Can you work these out from the model? Positions are in its coordinate system, mm. A direction names the side the tool comes from. Give positions to 0.01 mm unless a question says otherwise; leave off trailing zeros. Order: outer loops, then holes, each group sorted by start corner. A loop starts at its lowest first (then second) coordinate and runs counter-clockwise, first axis right, second up. Notation, with made-up numbers: M 2,88.5 L 46,88.5 A22 cw 46,104.5 Z; hole C -19.5,56.25 d10. An arc over 180 degrees is marked long. Use a Markdown table: item, result. Add a question column.
from build123d import *

# Parameters (mm, degrees)
SKETCH4_R                = 6.35
BOSS_EXTRUDE1_DEPTH      = 6.35
BOSS_EXTRUDE1_DEPTH_BACK = 6.35
SKETCH5_R                = 6.35
SKETCH5_R_2              = 5.9436
CUT_EXTRUDE1_DEPTH       = 1.4224
SKETCH7_W                = 1.89865
SKETCH7_H                = 6.35


with BuildPart() as part:
    # Sketch4 → Boss-Extrude1 (new body, two sides)
    with BuildSketch(Plane.XY.offset(39.04234)) as boss_extrude1_sk:
        with Locations((-94.293901082, 0)):
            Circle(SKETCH4_R)
    extrude(amount=BOSS_EXTRUDE1_DEPTH)
    extrude(boss_extrude1_sk.sketch, amount=-BOSS_EXTRUDE1_DEPTH_BACK)

    # Sketch5 → Cut-Extrude1 (cut)
    with BuildSketch(Plane.XY.offset(34.44494)):
        with Locations((-94.293901082, 0)):
            Circle(SKETCH5_R)
        with Locations((-94.293901082, 0)):
            Circle(SKETCH5_R_2, mode=Mode.SUBTRACT)
    extrude(amount=CUT_EXTRUDE1_DEPTH, mode=Mode.SUBTRACT)

    # Sketch7 → Tap Drill for _10-24 Tap1 (revolve, cut)
    with BuildSketch(Plane(origin=(-94.293901082, 0, 39.04234), x_dir=(0, 1, 0), z_dir=(1, 0, 0))):
        with Locations((0.949325, 3.175)):
            Rectangle(SKETCH7_W, SKETCH7_H)
    revolve(axis=Axis((-94.293901082, 0, 32.69234), (0, 0, 1)), mode=Mode.SUBTRACT)


solid = part.part
1. If we section it at D-D, the plane z = 42.75: List the corners of the cut face in (x, y) for me.
2. I need wall thicknesses on L1, parallel to Z at x = -95.5, y = 1; L2, parallel to X at y = 0.5, z = 41; L3, parallel to Y at x = -95, z = 41.5. Which ranges of each line are inside material? Lowest first, please. Write a range as [from, to].
3. Will these pins go through, and if not, where does the flat tip stop? pin 1 (3 mm diameter, centred on x = -98.5, y = -5, fed in from -Z); pin 2 (1 mm diameter, centred on y = -2.5, z = 44, fed in from +X); pin 3 (1 mm diameter, centred on y = -4, z = 40, fed in from +X); pin 4 (1.1 mm diameter, centred on x = -94, y = -1, fed in from +Z).
4. If we section it at A-A, the plane y = 0: List the corners of the cut face in (x, z) for me, then the cut area to 3 significant figures.
5. If we section it at B-B, the plane z = 36.25: List the corners of the cut face in (x, y) for me.
6. We'd pull the mould along Z, two halves only. Please class faces 1 (the face through (-94, 0, 32.692)), 2 (the face through (-99, -4, 34.445)), 3 (the face through (-88.24, 1.91, 40.7)): +Z half, -Z half, draft (parallel to the pull), parting line (faces both ways), or undercut.
7. On a 3-axis mill with a long thin cutter (end or side, diameter ignored), from which of +Z, -Z, +X, -X, +Y, -Y can I reach the whole of each face in a straight line? I mean faces 4 (the face through (-88.24, 1.91, 33.58)), 5 (the face through (-88.625, 1.785, 35.146)), 6 (the face through (-92.44, -0.41, 42.26)). Say none if no direction works.
8. If we section it at C-C, the plane x = -98: List the corners of the cut face in (y, z) for me, then the cut area to 3 significant figures.
Geometry results:
| question | item | result |
|---|---|---|
| 1 | outline | C -94.29,0 d12.7; hole C -94.29,0 d3.8 |
| 2 | L1 | z = [32.69, 39.04] |
| 2 | L2 | x = [-100.62, -96.13], [-92.46, -87.96] |
| 2 | L3 | y = [-6.31, -1.76], [1.76, 6.31] |
| 3 | pin 1 | stops at z = 32.69 |
| 3 | pin 2 | stops at x = -88.27 |
| 3 | pin 3 | stops at x = -89 |
| 3 | pin 4 | stops at z = 39.04 |
| 4 | outline | M -100.64,32.69 L -87.94,32.69 L -87.94,34.44 L -88.35,34.44 L -88.35,35.87 L -87.94,35.87 L -87.94,45.39 L -92.4,45.39 L -92.4,39.04 L -96.19,39.04 L -96.19,45.39 L -100.64,45.39 L -100.64,35.87 L -100.24,35.87 L -100.24,34.44 L -100.64,34.44 Z |
| 4 | area | 136 mm^2 |
| 5 | outline | C -94.29,0 d12.7 |
| 6 | face 1 | -Z half |
| 6 | face 2 | undercut |
| 6 | face 3 | draft |
| 7 | face 4 | +Z, -Z |
| 7 | face 5 | none |
| 7 | face 6 | +Z |
| 8 | outline | M -5.16,32.69 L 5.16,32.69 L 5.16,34.44 L 4.65,34.44 L 4.65,35.87 L 5.16,35.87 L 5.16,45.39 L -5.16,45.39 L -5.16,35.87 L -4.65,35.87 L -4.65,34.44 L -5.16,34.44 Z |
| 8 | area | 130 mm^2 |
